Verification items for the finished model (mm, model axes). A direction names the side the tool comes from. Give positions to 0.01 mm unless a question says otherwise; leave off trailing zeros. Write each loop counter-clockwise with the first axis right and the second up, starting at its lowest first coordinate (ties: lowest second). Pieces come first, ordered by that corner, then holes. Notation, with made-up numbers: (-20.5, 47) -> (8.5, 47) arc R12 ccw to (8.5, 57) -> close; hole circle Ø4 at (-19, -31). An arc over 180 degrees is marked (long way). Answer as CSV lines item,"result". Start each with the question number.
1) Material ranges on L1, parallel to X at y = 20, z = 7; L2, parallel to Y at x = 0.15, z = 10; L3, parallel to X at y = 8.5, z = 2.5, recorded low to high.
2) Gauge pin test, flat ends, axial feed: pin 1 Ø1.8 at (x, z) = (4.5, 1) entering from -Y; pin 2 Ø5 at (y, z) = (5, 10) entering from -X; pin 3 Ø4 at (x, z) = (5, 10.5) entering from +Y. Record the tip position at first contact, or that the pin passes through.
3) Sectioned sample at D-D on z = 17.25. Record the cut outline in (x, y).
4) Tool access check on faces 4 (the flat face through (-4, 8.42, 1)), 5 (the flat face through (4, 8.42, 1)), 6 (the flat face through (-2.5, 8, 10)), 7 (the flat face through (2.5, 9, 10)), 8 (the flat face through (5, 25, 10)). Record the directions out of +Z, -Z, +X, -X, +Y, -Y that give a thin tool (end or side, any length) a straight path to the whole face; none if there is none.
5) Sectioned sample at B-B on z = 11.5. Record the cut outline in (x, y), and give its area (3 significant figures).
6) Sectioned sample at C-C on x = 6. Record the cut outline in (y, z).
7) Mould release check, pull along Z, two halves, no side actions. Record for faces 1 (the flat face through (0, 19, 20)), 2 (the flat face through (0, 19.688, 10)), 3 (the cylindrical face through (-4, 14, 10)): released by +Z, released by -Z, zero draft, split by the parting line, or undercut.
8) Sectioned sample at A-A on y = 5. Record the cut outline in (x, z).
```python
from build123d import *

# Parameters (mm, degrees)
SALIENTE_EXTRUIR1_DEPTH = 20
CROQUIS2_R              = 2
CORTAR_EXTRUIR1_DEPTH   = 39.160843806
SALIENTE_EXTRUIR3_DEPTH = 4
CORTAR_EXTRUIR3_START   = -5
CORTAR_EXTRUIR3_DEPTH   = 5


# Read off the part's stored shape, not the designer's step: Cortar-Extruir3
with BuildPart() as part:
    # Croquis1 → Saliente-Extruir1 (new body)
    with BuildSketch(Plane.XY):
        Polygon((2.5, 0), (-2.5, 0), (-2.5, 15), (-10, 15), (-10, 30), (-0.771012727, 20.771012727), (-0.771012727, 19.688176129), (0.771012727, 19.688176129), (0.771012727, 20.771012727), (10, 30), (10, 15), (2.5, 15), align=None)
    extrude(amount=SALIENTE_EXTRUIR1_DEPTH)

    # Croquis2 → Cortar-Extruir1 (cut, through all)
    with BuildSketch(Plane.ZY.offset(2.5)):
        with Locations((10, 5)):
            Circle(CROQUIS2_R)
    extrude(amount=-CORTAR_EXTRUIR1_DEPTH, mode=Mode.SUBTRACT)

    # Croquis3 → Saliente-Extruir3 (add)
    with BuildSketch(Plane.ZY.offset(2.5)):
        with BuildLine():
            Line((0, 8.420482436), (0, 15))
            Line((0, 15), (20, 15))
            Line((20, 15), (20, 8.420482436))
            Line((20, 8.420482436), (18.324680168, 8.420482436))
            ThreePointArc((18.324680168, 8.420482436), (10, 14), (1.675319832, 8.420482436))
            Line((1.675319832, 8.420482436), (0, 8.420482436))
        make_face()
    saliente_extruir3 = extrude(amount=SALIENTE_EXTRUIR3_DEPTH)

    # Simetr_a2: Saliente-Extruir3 across plane
    add(saliente_extruir3.mirror(Plane.ZY))

    # Cortar-Extruir3 outline → Cortar-Extruir3 (cut)
    with BuildSketch(Plane.ZY.offset(2.5).offset(CORTAR_EXTRUIR3_START)):
        with BuildLine():
            ThreePointArc((20, 8.420482436), (16.536522861, 2.385496766), (10, 0))
            Line((10, 0), (20, 0))
            Line((20, 0), (20, 8.420482436))
        make_face()
        with BuildLine():
            ThreePointArc((10, 0), (3.463477139, 2.385496766), (0, 8.420482436))
            Line((0, 8.420482436), (0, 0))
            Line((0, 0), (10, 0))
        make_face()
    extrude(amount=CORTAR_EXTRUIR3_DEPTH, mode=Mode.SUBTRACT)


solid = part.part
```
Ans:
1,L1,"x = -10 to -0.77, 0.77 to 10"
1,L2,"y = 0 to 3, 7 to 19.69"
1,L3,"x = -2.5 to 2.5"
2,pin 1,"stops at y = 8.42"
2,pin 2,"stops at x = -2.5"
2,pin 3,"stops at y = 27"
3,outline,"(-10, 15) -> (-6.5, 15) -> (-6.5, 10.33) -> (-2.5, 10.33) -> (-2.5, 3.05) -> (2.5, 3.05) -> (2.5, 10.33) -> (6.5, 10.33) -> (6.5, 15) -> (10, 15) -> (10, 30) -> (0.77, 20.77) -> (0.77, 19.69) -> (-0.77, 19.69) -> (-0.77, 20.77) -> (-10, 30) -> close"
4,face 4,"+Z, -Z, -X, -Y"
4,face 5,"+Z, -Z, +X, -Y"
4,face 6,"-X, -Y"
4,face 7,"+X, -Y"
4,face 8,"+Z, -Z, +Y"
5,outline,"(-10, 15) -> (-6.5, 15) -> (-6.5, 13.87) -> (-2.5, 13.87) -> (-2.5, 6.32) -> (2.5, 6.32) -> (2.5, 13.87) -> (6.5, 13.87) -> (6.5, 15) -> (10, 15) -> (10, 30) -> (0.77, 20.77) -> (0.77, 19.69) -> (-0.77, 19.69) -> (-0.77, 20.77) -> (-10, 30) -> close; (-2.5, 0.11) -> (2.5, 0.11) -> (2.5, 3.68) -> (-2.5, 3.68) -> close"
5,area,"269 mm²"
6,outline,"(8.42, 0) -> (26, 0) -> (26, 20) -> (8.42, 20) -> (8.42, 18.32) arc R9 cw to (8.42, 1.68) -> close"
7,face 1,"released by +Z"
7,face 2,"zero draft"
7,face 3,"undercut"
8,outline,"(-2.5, 1.25) -> (2.5, 1.25) -> (2.5, 8) -> (-2.5, 8) -> close; (-2.5, 12) -> (2.5, 12) -> (2.5, 18.75) -> (-2.5, 18.75) -> close"
